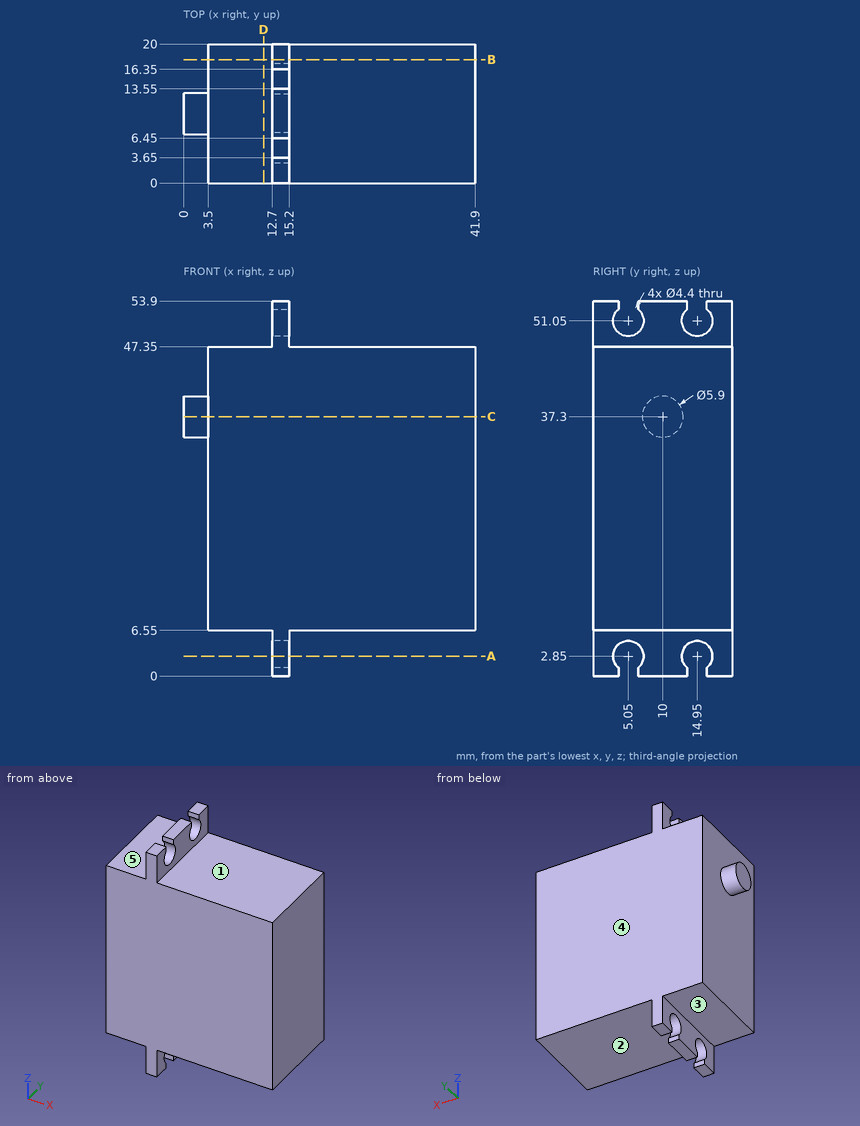
Part print with two shaded views. Sizes in mm from the minimum x, y, z corner. A direction names the side the tool comes from. Coordinates: 2 decimals unless noted, no trailing zeros. Write each loop counter-clockwise with the first axis right and the second up, starting at its lowest first coordinate (ties: lowest second). Pieces come first, ordered by that corner, then holes. Notation, with made-up numbers: (-28.75, 29) -> (25.25, 29) arc R10 ccw to (25.25, 43) -> close; hole circle Ø6 at (16, 16). An arc over 180 degrees is marked (long way). Return JSON: item names as keys, results as strings. Group by question number.
Q1. Cut at D-D, the plane x = 11.5. Give the cut face in (y, z), then the cut area to 3 significant figures.
Q2. Cut at A-A, the plane z = 2.85. Give the cut face in (x, y).
Q3. Cut at C-C, the plane z = 37.3. Give the cut face in (x, y).
Q4. Drill centre lines: line 1 (Y direction, x = 14.2, z = 2.85); line 2 (Y direction, x = 14, z = 2); line 3 (Z direction, x = 13.4, y = 5.05). Where is each one in solid material? Low to high.
Q5. Flat gauge pins, fed straight in: pin 1 (6 mm diameter, centred on y = 2, z = 19.5, fed in from -X); pin 2 (7 mm diameter, centred on y = 14.95, z = 2.85, fed in from -X); pin 3 (1.5 mm diameter, centred on x = 23.5, y = 3, fed in from -Z). Where does each tip first touch, or does it go through?
Q6. Which spindle directions (+Z, -Z, +X, -X, +Y, -Y) get a long thin tool onto all of the face, cutting with end or side? Do the marked faces 1, 2, 3, 4 and 5. Say none if no direction does.
Q7. Cut at B-B, the plane y = 17.75. Give the cut face in (x, z), then the cut area to 3 significant figures.
Returned:
{
 "1": {"outline": "(0, 6.55) -> (20, 6.55) -> (20, 47.35) -> (0, 47.35) -> close", "area": "816 mm2"},
 "2": {"outline": "(12.7, 0) -> (15.2, 0) -> (15.2, 2.85) -> (12.7, 2.85) -> close; (12.7, 7.25) -> (15.2, 7.25) -> (15.2, 12.75) -> (12.7, 12.75) -> close; (12.7, 17.15) -> (15.2, 17.15) -> (15.2, 20) -> (12.7, 20) -> close"},
 "3": {"outline": "(0, 7.05) -> (3.5, 7.05) -> (3.5, 0) -> (41.9, 0) -> (41.9, 20) -> (3.5, 20) -> (3.5, 12.95) -> (0, 12.95) -> close"},
 "4": {"line 1": "y = 0 to 2.85, 7.25 to 12.75, 17.15 to 20", "line 2": "y = 0 to 3.02, 7.08 to 12.92, 16.98 to 20", "line 3": "z = 5.05 to 48.85"},
 "5": {"pin 1": "stops at x = 3.5", "pin 2": "stops at x = 12.7", "pin 3": "stops at z = 6.55"},
 "6": {"face 1": "+Z, +X, +Y, -Y", "face 2": "-Z, +X, +Y, -Y", "face 3": "-Z, -X, +Y, -Y", "face 4": "+Z, -Z, +X, -X, +Y", "face 5": "+Z, -X, +Y, -Y"},
 "7": {"outline": "(3.5, 6.55) -> (12.7, 6.55) -> (12.7, 0) -> (15.2, 0) -> (15.2, 6.55) -> (41.9, 6.55) -> (41.9, 47.35) -> (15.2, 47.35) -> (15.2, 53.9) -> (12.7, 53.9) -> (12.7, 47.35) -> (3.5, 47.35) -> close", "area": "1,600 mm2"}
}
